Read the model definition and answer for the solid it produces. Units are mm, in the model's axes. A direction names the side the tool comes from. Coordinates: 2 decimals unless noted, no trailing zeros. Order: outer loops, then holes, each group sorted by start corner. A loop starts at its lowest first (then second) coordinate and runs counter-clockwise, first axis right, second up. Notation, with made-up numbers: M 62,18 L 80,18 A27 ccw 80,36 Z; hole C 80.5,12.5 d3. An arc over 180 degrees is marked long. Write each question's results on one line, items separated by ' | '.
```python
from build123d import *

# Parameters (mm, degrees)
F1_DEPTH = 2
F2_R     = 7.5
F3_DEPTH = 70
F6_W     = 65
F6_H     = 47
F7_DEPTH = 41.2
F8_R     = 6
F9_DEPTH = 12.8


with BuildPart() as f1:
    # F0 (on Top) → F1 (new body)
    with BuildSketch(Plane.XY):
        with BuildLine():
            Line((-42.7, -31.65), (42.7, -31.65))
            ThreePointArc((42.7, -31.65), (46.235534, -30.185534), (47.7, -26.65))
            Line((47.7, -26.65), (47.7, 26.65))
            ThreePointArc((47.7, 26.65), (46.235534, 30.185534), (42.7, 31.65))
            Line((42.7, 31.65), (-42.7, 31.65))
            ThreePointArc((-42.7, 31.65), (-46.235534, 30.185534), (-47.7, 26.65))
            Line((-47.7, 26.65), (-47.7, -26.65))
            ThreePointArc((-47.7, -26.65), (-46.235534, -30.185534), (-42.7, -31.65))
        make_face()
        with BuildLine():
            Line((-41.5, -26.078427), (-41.5, -20.421573))
            ThreePointArc((-41.5, -20.421573), (-38, -18.75), (-34.5, -20.421573))
            Line((-34.5, -20.421573), (-34.5, -26.078427))
            ThreePointArc((-34.5, -26.078427), (-38, -27.75), (-41.5, -26.078427))
        make_face(mode=Mode.SUBTRACT)
        with BuildLine():
            ThreePointArc((34.5, -20.421573), (38, -18.75), (41.5, -20.421573))
            Line((41.5, -20.421573), (41.5, -26.078427))
            ThreePointArc((41.5, -26.078427), (38, -27.75), (34.5, -26.078427))
            Line((34.5, -26.078427), (34.5, -20.421573))
        make_face(mode=Mode.SUBTRACT)
        with BuildLine():
            ThreePointArc((-34.203752, 2.65), (-33.2, 0), (-34.203752, -2.65))
            Line((-34.203752, -2.65), (-40.196248, -2.65))
            ThreePointArc((-40.196248, -2.65), (-41.2, 0), (-40.196248, 2.65))
            Line((-40.196248, 2.65), (-34.203752, 2.65))
        make_face(mode=Mode.SUBTRACT)
        with BuildLine():
            ThreePointArc((-41.5, 26.078427), (-38, 27.75), (-34.5, 26.078427))
            Line((-34.5, 26.078427), (-34.5, 20.421573))
            ThreePointArc((-34.5, 20.421573), (-38, 18.75), (-41.5, 20.421573))
            Line((-41.5, 20.421573), (-41.5, 26.078427))
        make_face(mode=Mode.SUBTRACT)
        with BuildLine():
            ThreePointArc((34.203752, -2.65), (33.2, 0), (34.203752, 2.65))
            Line((34.203752, 2.65), (40.196248, 2.65))
            ThreePointArc((40.196248, 2.65), (41.2, 0), (40.196248, -2.65))
            Line((40.196248, -2.65), (34.203752, -2.65))
        make_face(mode=Mode.SUBTRACT)
        with BuildLine():
            Line((41.5, 26.078427), (41.5, 20.421573))
            ThreePointArc((41.5, 20.421573), (38, 18.75), (34.5, 20.421573))
            Line((34.5, 20.421573), (34.5, 26.078427))
            ThreePointArc((34.5, 26.078427), (38, 27.75), (41.5, 26.078427))
        make_face(mode=Mode.SUBTRACT)
    extrude(amount=-F1_DEPTH)

    # F2 (on face) → F3 (join)
    with BuildSketch(Plane.XY):
        Circle(F2_R)
    extrude(amount=F3_DEPTH)

    # F4 (on Front) → F5 (revolve)
    with BuildSketch(Plane.XZ):
        with BuildLine():
            ThreePointArc((0, 74.590989), (-11.667262, 69.758251), (-16.5, 58.090989))
            ThreePointArc((-16.5, 58.090989), (-16.499956, 58.063064), (-16.499905, 58.03514))
            ThreePointArc((-16.499905, 58.03514), (-14.834915, 39.084766), (-9.962409, 20.695977))
            Line((-9.962409, 20.695977), (0, 20.695977))
            Line((0, 20.695977), (0, 74.590989))
        make_face()
    revolve(axis=Axis((0, 0, 47.643483), (0, 0, -1)))

    # F6 (on face) → F7 (join)
    with BuildSketch(Plane(origin=(0, 0, -2), x_dir=(1, 0, 0), z_dir=(0, 0, -1))):
        Rectangle(F6_W, F6_H)
    extrude(amount=F7_DEPTH)

    # F8 (on face) → F9 (join)
    with BuildSketch(Plane(origin=(0, 0, -43.2), x_dir=(1, 0, 0), z_dir=(0, 0, -1))):
        Circle(F8_R)
    extrude(amount=F9_DEPTH)


solid = f1.part
```
(1) The part is cut by section A-A, the plane y = -22. Write down the section's boundary in (x, z), then the cut area to 3 significant figures.
Conclusion:
outline: M -47.7,-2 L -41.5,-2 L -41.5,0 L -47.7,0 Z; M -34.5,-2 L -32.5,-2 L -32.5,-43.2 L 32.5,-43.2 L 32.5,-2 L 34.5,-2 L 34.5,0 L -34.5,0 Z; M 41.5,-2 L 47.7,-2 L 47.7,0 L 41.5,0 Z | area: 2,840 mm²
(2) Straight lines are drawn through the part: line 1 (X direction, y = 3, z = -21); line 2 (Y direction, x = 30, z = -13); line 3 (Z direction, x = -4.5, y = 24.5). For each, find the intervals that lie inside material, in ascending order.
Conclusion:
line 1: -32.5 to 32.5 | line 2: -23.5 to 23.5 | line 3: -2 to 0
(3) The part is cut by section C-C, the plane z = -21.5. Write down the section's boundary in (x, y).
Conclusion:
outline: M -32.5,-23.5 L 32.5,-23.5 L 32.5,23.5 L -32.5,23.5 Z
(4) For faces 1 (the flat face through (-32.5, 0, -22)), 2 (the flat face through (0, -23.5, -22)), 3 (the flat face through (32.5, 0, -22)), determine the directions among +Z, -Z, +X, -X, +Y, -Y from which every point of the face is accessible in a straight line to the end or side of a thin tool.
Conclusion:
face 1: -Z, -X, +Y, -Y | face 2: -Z, +X, -X, -Y | face 3: -Z, +X, +Y, -Y
(5) The mould has two halves that part along Z. Classify faces 4 (the flat face through (4, 7, 20.696)), 5 (the cylindrical face through (46.27, 30.15, -0.99)), 6 (the flat face through (-8, 0, -43.2)), 7 (the cylindrical face through (-7.493, 0.33, 10.203)): pulls with the +Z half, pulls with the -Z half, needs draft (parallel to the pull), parting line crosses it, or undercut.
Conclusion:
face 4: undercut | face 5: needs draft | face 6: pulls with the -Z half | face 7: undercut
(6) The part is cut by section B-B, the plane x = 27.5. Write down the section's boundary in (y, z), then the cut area to 3 significant figures.
Conclusion:
outline: M -31.65,-2 L -23.5,-2 L -23.5,-43.2 L 23.5,-43.2 L 23.5,-2 L 31.65,-2 L 31.65,0 L -31.65,0 Z | area: 2,060 mm²
(7) Given pin 1 (12 mm diameter, centred on y = 20.5, z = 23.5, fed in from -X); pin 2 (2 mm diameter, centred on x = 7, z = -12, fed in from -Y); pin 3 (2 mm diameter, centred on x = -14.5, z = -3.5, fed in from +Y); pin 4 (12 mm diameter, centred on x = 14, y = 13, fed in from +Z), each flat-ended and moving along its own axis, determine where each tip first touches the part or whether it passes through.
Conclusion:
pin 1: through | pin 2: y = -23.5 | pin 3: y = 23.5 | pin 4: z = 68.12
